```python
from build123d import *

# Parameters (mm, degrees)
SKETCH1_R           = 100
SKETCH1_R_2         = 2.1
SKETCH1_R_3         = 1.27
BOSS_EXTRUDE1_DEPTH = 3.175


with BuildPart() as part:
    # Sketch1 → Boss-Extrude1 (new body)
    with BuildSketch(Plane(origin=(0, 0, 0), x_dir=(1, 0, 0), z_dir=(0, 1, 0))):
        with Locations(Location((0, 0, 0), (0, 0, 270))):
            Circle(SKETCH1_R)
        with Locations(Location((24.32899024, 90.797027671, 0), (0, 0, 270))):
            Circle(SKETCH1_R_2, mode=Mode.SUBTRACT)
        with Locations(Location((-24.32899024, 90.797027671, 0), (0, 0, 90))):
            Circle(SKETCH1_R_2, mode=Mode.SUBTRACT)
        with Locations(Location((90.797027671, -24.32899024, 0), (0, 0, 90))):
            Circle(SKETCH1_R_2, mode=Mode.SUBTRACT)
        with Locations(Location((66.468037432, -66.468037432, 0), (0, 0, 270))):
            Circle(SKETCH1_R_2, mode=Mode.SUBTRACT)
        with Locations(Location((-66.468037432, -66.468037432, 0), (0, 0, 90))):
            Circle(SKETCH1_R_2, mode=Mode.SUBTRACT)
        with Locations(Location((-90.797027671, -24.32899024, 0), (0, 0, 270))):
            Circle(SKETCH1_R_2, mode=Mode.SUBTRACT)
        with Locations(Location((-10.16, 7.62, 0), (0, 0, 270))):
            Circle(SKETCH1_R_3, mode=Mode.SUBTRACT)
        with Locations(Location((-10.16, -7.62, 0), (0, 0, 270))):
            Circle(SKETCH1_R_3, mode=Mode.SUBTRACT)
        with Locations(Location((10.16, -7.62, 0), (0, 0, 270))):
            Circle(SKETCH1_R_3, mode=Mode.SUBTRACT)
        with Locations(Location((10.16, 7.62, 0), (0, 0, 270))):
            Circle(SKETCH1_R_3, mode=Mode.SUBTRACT)
        with Locations(Location((25.16, 6.35, 0), (0, 0, 270))):
            Circle(SKETCH1_R_3, mode=Mode.SUBTRACT)
        with Locations(Location((25.16, -6.35, 0), (0, 0, 270))):
            Circle(SKETCH1_R_3, mode=Mode.SUBTRACT)
        with Locations(Location((45.48, -6.35, 0), (0, 0, 270))):
            Circle(SKETCH1_R_3, mode=Mode.SUBTRACT)
        with Locations(Location((45.48, 6.35, 0), (0, 0, 270))):
            Circle(SKETCH1_R_3, mode=Mode.SUBTRACT)
        with Locations(Location((-45.48, 6.35, 0), (0, 0, 90))):
            Circle(SKETCH1_R_3, mode=Mode.SUBTRACT)
        with Locations(Location((-45.48, -6.35, 0), (0, 0, 90))):
            Circle(SKETCH1_R_3, mode=Mode.SUBTRACT)
        with Locations(Location((-25.16, -6.35, 0), (0, 0, 90))):
            Circle(SKETCH1_R_3, mode=Mode.SUBTRACT)
        with Locations(Location((-25.16, 6.35, 0), (0, 0, 90))):
            Circle(SKETCH1_R_3, mode=Mode.SUBTRACT)
    extrude(amount=BOSS_EXTRUDE1_DEPTH)


solid = part.part
```
Could you check a few things on this model? Use its own coordinates, in mm. Round coordinates to 2 decimals unless told otherwise and drop trailing zeros. Order: outer loops, then holes, each group sorted by start corner. A loop starts at its lowest first (then second) coordinate and runs counter-clockwise, first axis right, second up. Notation, with made-up numbers: (79.25, -33.5) -> (119.25, -33.5) arc R27 ccw to (119.25, -8.5) -> close; hole circle Ø6 at (-24, 12.5). An arc over 180 degrees is marked (long way). One line per question, with ' | ' between items.
Q1. I'm going to push a flat-ended pin straight in: pin 1 (1.5 mm diameter, centred on x = -45.48, z = -6.35, fed in from -Y). Where does the tip first touch, or does it pass through?
Computed values:
pin 1: through
Q2. If we section it at B-B on x = 75.5: Write out the boundary of the cut face in (y, z) (3 decimals), plus the area to 3 significant figures.
Computed values:
outline: (0, -65.572) -> (3.175, -65.572) -> (3.175, 65.572) -> (0, 65.572) -> close | area: 416 mm²
Q3. If we section it at A-A on y = 2.2: Give the number of separate pieces and of enclosed holes in the cut face, plus the area to 3 significant figures.
Computed values:
separate pieces: 1 | enclosed holes: 18 | area: 31,300 mm²
Q4. If we section it at C-C on z = -68: Write out the boundary of the cut face in (x, y) (3 decimals), plus the area to 3 significant figures.
Computed values:
outline: (-73.321, 0) -> (73.321, 0) -> (73.321, 3.175) -> (-73.321, 3.175) -> close | area: 466 mm²
Q5. If I drill on line 1 (Z direction, x = -45, y = 2.35); line 2 (X direction, y = 1.35, z = 66); line 3 (X direction, y = 1.1, z = 4), over which ranges is the centre line in solid material (lowest first)? Write a range as from..to.
Computed values:
line 1: -89.3..-7.53, -5.17..5.17, 7.53..89.3 | line 2: -75.13..-68.52, -64.42..64.42, 68.52..75.13 | line 3: -99.92..99.92
